Read the model definition and answer for the solid it produces. Units are mm, in the model's axes. A direction names the side the tool comes from. Round coordinates to 2 decimals unless told otherwise and drop trailing zeros. Order: outer loops, then holes, each group sorted by start corner. A loop starts at its lowest first (then second) coordinate and runs counter-clockwise, first axis right, second up. Notation, with made-up numbers: (53.25, 4) -> (106.25, 4) arc R22 cw to (106.25, 33) -> close; hole circle Ø11 at (-5.5, -0.75). An arc over 180 degrees is marked (long way). Answer as a JSON object with one key per item and string values. Group by question number.
Item 1: Section A-A, the plane y = 2.5 is taken. Write down the section's boundary in (x, z), plus the area to 3 significant figures.
Item 2: Section B-B, the plane x = 0 is taken. Write down the section's boundary in (y, z), plus the area to 3 significant figures.
Item 3: Consider probe 1 along X at (y, z) = (16.5, 7); probe 2 along Z at (x, y) = (0, -10); probe 3 along Z at (x, y) = (-33.5, 26.5). Determine where each line is inside the solid, lowest interval first. Write a range as from..to.
Item 4: Section D-D, the plane z = 7 is taken. Write down the section's boundary in (x, y), plus the area to 3 significant figures.
Item 5: The mould has two halves that part along Y. Classify faces 3 (the flat face through (0, -11, -15)), 4 (the flat face through (0, 0, 4)), 5 (the cylindrical face through (34, 25.5, 0)): pulls with the +Y half, pulls with the -Y half, needs draft (parallel to the pull), parting line crosses it, or undercut.
Item 6: For faces 1 (the cylindrical face through (-34, 27.5, 0)), 2 (the flat face through (-33, 20, 0)), determine the directions among +Z, -Z, +X, -X, +Y, -Y from which every point of the face is accessible in a straight line to the end or side of a thin tool.
Item 7: Given P1, Ø3, axis at x = 0, z = 0, coming from the +Y side, flat-ended and moving along its own axis, determine where the tip first touches the part or whether it passes through.
Item 8: Section C-C, the plane y = 26.5 is taken. Write down the section's boundary in (x, z), plus the area to 3 significant figures.
from build123d import *

# Parameters (mm, degrees)
F0_W     = 2
F0_H     = 30
F0_W_2   = 66
F0_R     = 1
F1_DEPTH = 25
F2_DEPTH = 25
F3_R     = 1
F4_DEPTH = 2
F5_R     = 1
F6_DEPTH = 2


# Not quite as in the source:
# - a feature names something its author has since deleted; it is built from what else it names


with BuildPart() as f1:
    # F0 (on Front) → F1 (new body)
    with BuildSketch(Plane.XZ):
        with Locations((-34, 0)):
            Rectangle(F0_W, F0_H)
        with Locations((34, 0)):
            Rectangle(F0_W, F0_H)
        Rectangle(F0_W_2, F0_H)
        Circle(F0_R, mode=Mode.SUBTRACT)
    extrude(amount=F1_DEPTH)

    # F0 (on Front) → F2 (join)
    with BuildSketch(Plane.XZ):
        with Locations((34, 0)):
            Rectangle(F0_W, F0_H)
        with Locations((-34, 0)):
            Rectangle(F0_W, F0_H)
    extrude(amount=-F2_DEPTH)

    # F3 (on face) → F4 (join)
    with BuildSketch(Plane.YZ.offset(35)):
        with BuildLine():
            Line((25, 15), (25, -15))
            ThreePointArc((25, -15), (40, 0), (25, 15))
        make_face()
        with Locations((26.5, 0)):
            Circle(F3_R, mode=Mode.SUBTRACT)
    extrude(amount=-F4_DEPTH)

    # F5 (on face) → F6 (join)
    with BuildSketch(Plane(origin=(-35, 0, 0), x_dir=(0, -1, 0), z_dir=(-1, 0, 0))):
        with BuildLine():
            Line((-25, -15), (-25, 15))
            ThreePointArc((-25, 15), (-40, 0), (-25, -15))
        make_face()
        with Locations((-26.5, 0)):
            Circle(F5_R, mode=Mode.SUBTRACT)
    extrude(amount=-F6_DEPTH)


solid = f1.part
Values found:
{
 "1": {"outline": "(-35, -15) -> (-33, -15) -> (-33, 15) -> (-35, 15) -> close; (33, -15) -> (35, -15) -> (35, 15) -> (33, 15) -> close", "area": "120 mm2"},
 "2": {"outline": "(-25, -15) -> (0, -15) -> (0, -1) -> (-25, -1) -> close; (-25, 1) -> (0, 1) -> (0, 15) -> (-25, 15) -> close", "area": "700 mm2"},
 "3": {"probe 1": "-35..-33, 33..35", "probe 2": "-15..-1, 1..15", "probe 3": "-14.92..-1, 1..14.92"},
 "4": {"outline": "(-35, -25) -> (35, -25) -> (35, 38.27) -> (33, 38.27) -> (33, 0) -> (-33, 0) -> (-33, 38.27) -> (-35, 38.27) -> close", "area": "1,900 mm2"},
 "5": {"face 3": "needs draft", "face 4": "pulls with the +Y half", "face 5": "undercut"},
 "6": {"face 1": "+X, -X", "face 2": "+Z, -Z, +Y"},
 "7": {"P1": "y = 0"},
 "8": {"outline": "(-35, -14.92) -> (-33, -14.92) -> (-33, -1) -> (-35, -1) -> close; (-35, 1) -> (-33, 1) -> (-33, 14.92) -> (-35, 14.92) -> close; (33, -14.92) -> (35, -14.92) -> (35, -1) -> (33, -1) -> close; (33, 1) -> (35, 1) -> (35, 14.92) -> (33, 14.92) -> close", "area": "111 mm2"}
}
